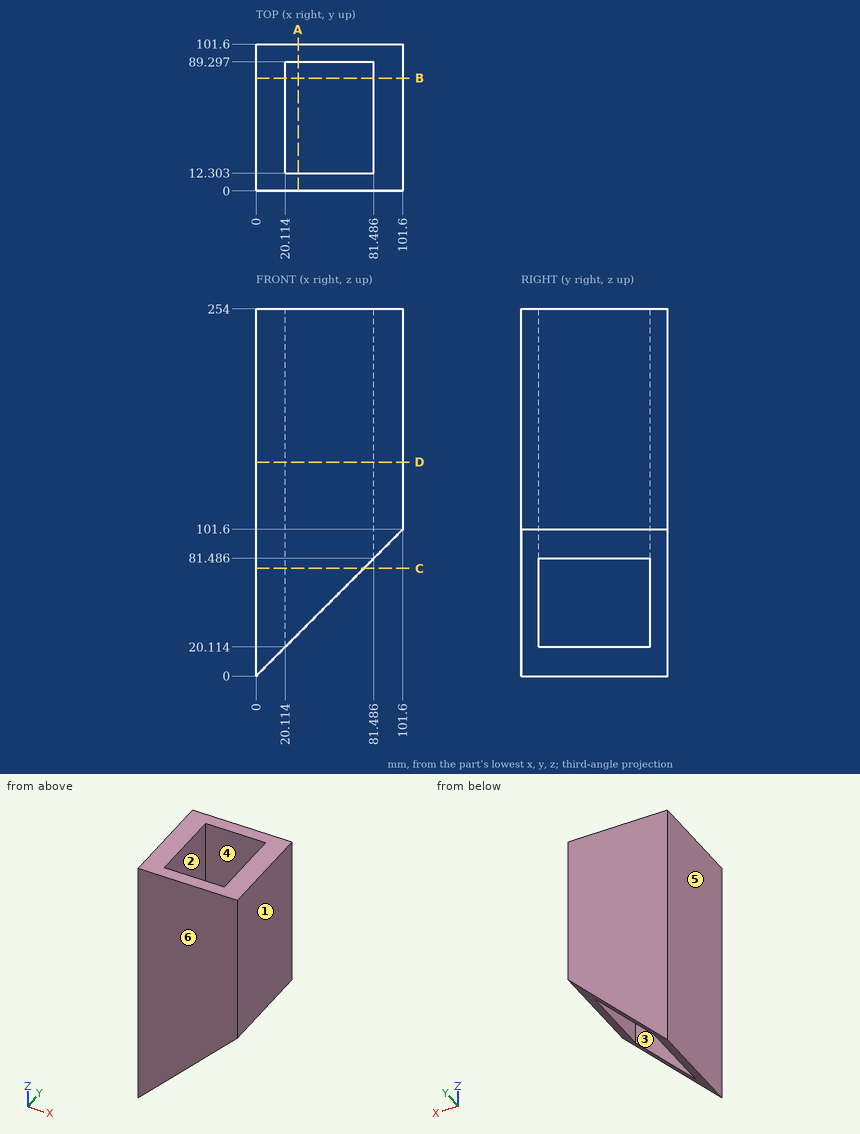
Print and shaded views of the part. All mm, measured from the part's lowest x, y and z. A direction names the side the tool comes from. Coordinates: 2 decimals unless noted, no trailing zeros. Order: outer loops, then holes, each group sorted by start corner. A loop starts at its lowest first (then second) coordinate and runs counter-clockwise, first axis right, second up.
Item 1: Saw through at B-B on y = 78. List the corners of the cut face in (x, z), then the cut area to 3 significant figures.
Filled in:
outline: (0, 0) - (20.11, 20.11) - (20.11, 254) - (0, 254) - close; (81.49, 81.49) - (101.6, 101.6) - (101.6, 254) - (81.49, 254) - close
area: 8,170 mm2
Item 2: Mould opens along X. For the marked faces 3, 4, 5 and 6 say: released by +X, released by -X, zero draft, split by the parting line, or undercut.
Filled in:
face 3: undercut
face 4: undercut
face 5: released by -X
face 6: zero draft
Item 3: Drill centre lines: L1, parallel to Y at x = 75.5, z = 218; L2, parallel to X at y = 29, z = 221.5; L3, parallel to X at y = 49.5, z = 82 (1 decimal). Where is each one in solid material? Low to high.
Filled in:
L1: y = 0 to 12.3, 89.3 to 101.6
L2: x = 0 to 20.11, 81.49 to 101.6
L3: x = 0 to 20.1, 81.5 to 82
Item 4: Saw through at A-A on x = 29. List the corners of the cut face in (y, z), then the cut area to 3 significant figures.
Filled in:
outline: (0, 29) - (12.3, 29) - (12.3, 254) - (0, 254) - close; (89.3, 29) - (101.6, 29) - (101.6, 254) - (89.3, 254) - close
area: 5,540 mm2
Item 5: Drop flat-ended pins along their axis: pin 1 Ø10 at (x, y) = (11.5, 38) entering from -Z; pin 2 Ø1.5 at (x, y) = (86.5, 23) entering from -Z; pin 3 Ø5 at (x, y) = (77, 67) entering from -Z; pin 4 Ø2 at (x, y) = (85.5, 89.5) entering from -Z. Give the stop position or say it passes through.
Filled in:
pin 1: stops at z = 6.5
pin 2: stops at z = 85.75
pin 3: passes through
pin 4: stops at z = 84.5
Item 6: Saw through at C-C on z = 74.5. List the corners of the cut face in (x, y), then the cut area to 3 significant figures.
Filled in:
outline: (0, 0) - (74.5, 0) - (74.5, 12.3) - (20.11, 12.3) - (20.11, 89.3) - (74.5, 89.3) - (74.5, 101.6) - (0, 101.6) - close
area: 3,380 mm2
Item 7: Saw through at D-D on z = 148. List the corners of the cut face in (x, y), then the cut area to 3 significant figures.
Filled in:
outline: (0, 0) - (101.6, 0) - (101.6, 101.6) - (0, 101.6) - close; hole (20.11, 12.3) - (81.49, 12.3) - (81.49, 89.3) - (20.11, 89.3) - close
area: 5,600 mm2
Item 8: Tool access for the marked faces 1 and 2: list every direction of +Z, -Z, +X, -X, +Y, -Y with a clear straight run to the whole face (end or side of a thin tool).
Filled in:
face 1: +Z, -Z, +X, +Y, -Y
face 2: +Z, -Z
